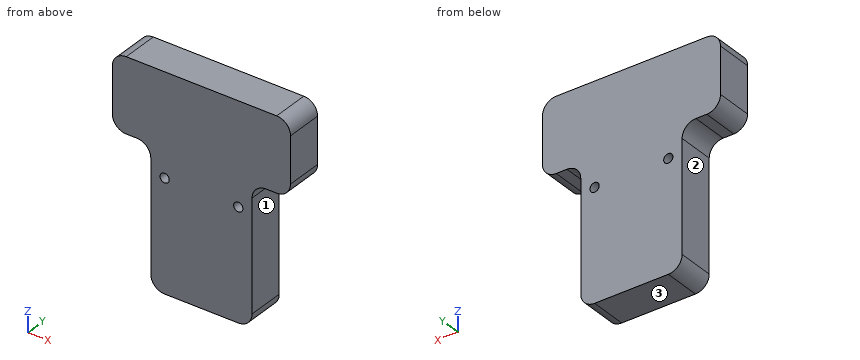
```python
from build123d import *

# Parameters (mm, degrees)
F0_R     = 1.5
F1_DEPTH = 12
F2_R     = 4.5


with BuildPart() as f1:
    # F0 (on Front) → F1 (new body)
    with BuildSketch(Plane.XZ):
        Polygon((-16.5, 9), (-16.5, -36), (16.5, -36), (16.5, 9), (29, 9), (29, 33), (-29, 33), (-29, 9), align=None)
        with Locations((-12, 0)):
            Circle(F0_R, mode=Mode.SUBTRACT)
        with Locations((12, 0)):
            Circle(F0_R, mode=Mode.SUBTRACT)
    extrude(amount=F1_DEPTH)

    # F2
    f2_edges = [f1.edges().sort_by_distance(p)[0] for p in [
        (-29, -6, 33),
        (-29, -6, 9),
        (-16.5, -6, 9),
        (-16.5, -6, -36),
        (16.5, -6, -36),
        (16.5, -6, 9),
        (29, -6, 9),
        (29, -6, 33),
    ]]
    fillet(f2_edges, radius=F2_R)


solid = f1.part
```
Geometry: final body of the model. Coordinates: model frame, mm. Face numbers are marked on the shaded views. A direction names the side the tool comes from. Give positions to 0.01 mm unless a question says otherwise; leave off trailing zeros. Order: outer loops, then holes, each group sorted by start corner. A loop starts at its lowest first (then second) coordinate and runs counter-clockwise, first axis right, second up. Notation, with made-up numbers: (38, 13.5) -> (76, 13.5) arc R18 cw to (76, 22.5) -> close; hole circle Ø8 at (38, -21.75). An arc over 180 degrees is marked (long way). Write each question's results on one line, items separated by ' | '. Start each with the question number.
1) Section A-A (z = 0). Return loops of the section in (x, y), then the cut area to 3 significant figures.
2) Set-up query: the marked faces 1, 2 and 3. Return all of +Z, -Z, +X, -X, +Y, -Y with unobstructed straight access to the full face (end or side cutting, diameter ignored); none if empty.
3) First-contact query: pin 1 (1 mm diameter, centred on x = 22.5, y = -3.5, fed in from -Z); pin 2 (5 mm diameter, centred on y = -4.5, z = 7, fed in from +X). Flat tips, straight axial feed; report the tip coordinate or a pass-through.
4) Section D-D (x = -23). Return loops of the section in (y, z).
5) Section C-C (z = -29). Return loops of the section in (x, y).
6) Line query: line 1 (Z direction, x = -12, y = -3.25); line 2 (Z direction, x = -24, y = -10); line 3 (X direction, y = -9.5, z = -30.5). Output: solid intervals per line, ascending. Write a range as from..to.
7) Section B-B (y = -1). Return loops of the section in (x, z).
Calculated:
1) outline: (-16.5, -12) -> (-13.5, -12) -> (-13.5, 0) -> (-16.5, 0) -> close; (-10.5, -12) -> (10.5, -12) -> (10.5, 0) -> (-10.5, 0) -> close; (13.5, -12) -> (16.5, -12) -> (16.5, 0) -> (13.5, 0) -> close | area: 324 mm2
2) face 1: -Z, +X, +Y, -Y | face 2: -Z, -X, +Y, -Y | face 3: -Z, +X, -X, +Y, -Y
3) pin 1: z = 9 | pin 2: x = 26.56
4) outline: (-12, 9) -> (0, 9) -> (0, 33) -> (-12, 33) -> close
5) outline: (-16.5, -12) -> (16.5, -12) -> (16.5, 0) -> (-16.5, 0) -> close
6) line 1: -36..-1.5, 1.5..33 | line 2: 9..33 | line 3: -16.5..16.5
7) outline: (-29, 13.5) arc R4.5 ccw to (-24.5, 9) -> (-21, 9) arc R4.5 cw to (-16.5, 4.5) -> (-16.5, -31.5) arc R4.5 ccw to (-12, -36) -> (12, -36) arc R4.5 ccw to (16.5, -31.5) -> (16.5, 4.5) arc R4.5 cw to (21, 9) -> (24.5, 9) arc R4.5 ccw to (29, 13.5) -> (29, 28.5) arc R4.5 ccw to (24.5, 33) -> (-24.5, 33) arc R4.5 ccw to (-29, 28.5) -> close; hole circle Ø3 at (-12, 0); hole circle Ø3 at (12, 0)
